Model file for the job. Use its own axes, mm. Face numbers are marked on the shaded views. A direction names the side the tool comes from. Round coordinates to 2 decimals unless told otherwise and drop trailing zeros. Order: outer loops, then holes, each group sorted by start corner. A loop starts at its lowest first (then second) coordinate and runs counter-clockwise, first axis right, second up. Notation, with made-up numbers: (25, -23) -> (30, -23) arc R15 ccw to (30, 3) -> close; hole circle Ø6 at (-20.5, 41.5). An arc over 180 degrees is marked (long way). Answer as CSV lines item,"result".
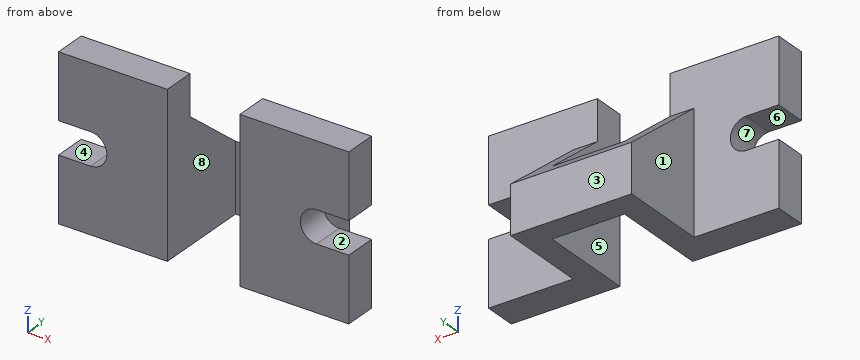
```python
from build123d import *

# Parameters (mm, degrees)
SKETCH_1_W               = 72
SKETCH_1_H               = 40
EXTRUDE_1_DEPTH          = 8
SKETCH_2_W               = 30
SKETCH_2_H               = 40
EXTRUDE_2_DEPTH          = 30
CUT_EXTRUDE_1_DEPTH      = 30
CUT_EXTRUDE_1_DEPTH_BACK = 30
CUT_EXTRUDE_2_DEPTH      = 30
CUT_EXTRUDE_2_DEPTH_BACK = 30
SKETCH_4_W               = 18
SKETCH_4_H               = 24
CUT_EXTRUDE_4_DEPTH      = 30
CUT_EXTRUDE_4_DEPTH_BACK = 30


with BuildPart() as part:
    # 草图1 → 凸台-拉伸1 (new body)
    with BuildSketch(Plane(origin=(0, 0, 0), x_dir=(1, 0, 0), z_dir=(0, 1, 0))):
        Rectangle(SKETCH_1_W, SKETCH_1_H)
    extrude(amount=EXTRUDE_1_DEPTH)

    # 草图2 → 凸台-拉伸2 (add)
    with BuildSketch(Plane(origin=(0, 0, 0), x_dir=(1, 0, 0), z_dir=(0, 1, 0))):
        Rectangle(SKETCH_2_W, SKETCH_2_H)
    extrude(amount=EXTRUDE_2_DEPTH)

    # 草图3 → 切除-拉伸1 (cut, two sides: drawn at the far end of the back side and taken through both)
    with BuildSketch(Plane(origin=(0, 0, 0), x_dir=(0, 0, -1), z_dir=(1, 0, 0)).offset(-CUT_EXTRUDE_1_DEPTH_BACK)):
        Polygon((-9.996476923, 8), (8, 30), (-20, 30), (-20, 8), align=None)
    extrude(amount=CUT_EXTRUDE_1_DEPTH + CUT_EXTRUDE_1_DEPTH_BACK, mode=Mode.SUBTRACT)

    # 草图4 → 切除-拉伸2 (cut, two sides: drawn at the far end of the back side and taken through both)
    with BuildSketch(Plane.XY.offset(-CUT_EXTRUDE_2_DEPTH_BACK)):
        with Locations((0, 12)):
            Rectangle(SKETCH_4_W, SKETCH_4_H)
    extrude(amount=CUT_EXTRUDE_2_DEPTH + CUT_EXTRUDE_2_DEPTH_BACK, mode=Mode.SUBTRACT)

    # 草图7 → 切除-拉伸4 (cut, two sides: drawn at the far end of the back side and taken through both)
    with BuildSketch(Plane(origin=(0, 0, 0), x_dir=(1, 0, 0), z_dir=(0, 1, 0)).offset(-CUT_EXTRUDE_4_DEPTH_BACK)):
        with BuildLine():
            Line((-28, 4), (-36, 4))
            Line((-36, 4), (-36, -4))
            Line((-36, -4), (-28, -4))
            ThreePointArc((-28, -4), (-24, 0), (-28, 4))
        make_face()
        with BuildLine():
            Line((28, 4), (36, 4))
            Line((36, 4), (36, -4))
            Line((36, -4), (28, -4))
            ThreePointArc((28, -4), (24, 0), (28, 4))
        make_face()
    extrude(amount=CUT_EXTRUDE_4_DEPTH + CUT_EXTRUDE_4_DEPTH_BACK, mode=Mode.SUBTRACT)


solid = part.part
```
Q1. Saw through at C-C (z = 8). Write the cut outline in (x, y), plus the area to 3 significant figures.
Checks:
outline,"(-36, 0) -> (-9, 0) -> (-9, 10.44) -> (-15, 10.44) -> (-15, 8) -> (-36, 8) -> close; (9, 0) -> (36, 0) -> (36, 8) -> (15, 8) -> (15, 10.44) -> (9, 10.44) -> close"
area,"461 mm²"
Q2. Saw through at A-A (y = 5.5). Write the cut outline in (x, z), plus the area to 3 significant figures.
Checks:
outline,"(-36, -20) -> (-9, -20) -> (-9, 20) -> (-36, 20) -> (-36, 4) -> (-28, 4) arc R4 cw to (-28, -4) -> (-36, -4) -> close; (9, -20) -> (36, -20) -> (36, -4) -> (28, -4) arc R4 cw to (28, 4) -> (36, 4) -> (36, 20) -> (9, 20) -> close"
area,"1,980 mm²"
Q3. Saw through at B-B (x = -31). Write the cut outline in (y, z).
Checks:
outline,"(0, -20) -> (8, -20) -> (8, -4) -> (0, -4) -> close; (0, 4) -> (8, 4) -> (8, 20) -> (0, 20) -> close"
Q4. Flat gauge pins, fed straight in: pin 1 (17.5 mm diameter, centred on y = 22, z = -4.5, fed in from -X); pin 2 (5 mm diameter, centred on x = -13.5, z = 16, fed in from +Y); pin 3 (1 mm diameter, centred on x = 10.5, z = 1.5, fed in from +Y). Where does each tip first touch, or does it go through?
Checks:
pin 1,"x = -15"
pin 2,"y = 8"
pin 3,"y = 19"
Q5. Mould opens along X. For the marked faces 6, 7 and 8 say: +X half, -X half, draft (parallel to the pull), parting line (faces both ways), or undercut.
Checks:
face 6,"draft"
face 7,"-X half"
face 8,"undercut"
Q6. Wall check: L1, parallel to X at y = 18.5, z = -16.5; L2, parallel to X at y = 4.5, z = 11.5; L3, parallel to Y at x = 26.5, z = -16. Give the ranges that are in metal, low to high. Write a range as [from, to].
Checks:
L1,"[-15, -9], [9, 15]"
L2,"[-36, -9], [9, 36]"
L3,"[0, 8]"
Q7. Saw through at D-D (z = -15). Write the cut outline in (x, y).
Checks:
outline,"(-36, 0) -> (-9, 0) -> (-9, 24) -> (9, 24) -> (9, 0) -> (36, 0) -> (36, 8) -> (15, 8) -> (15, 30) -> (-15, 30) -> (-15, 8) -> (-36, 8) -> close"
Q8. Tool access for the marked faces 1, 2, 3, 4 and 5: list every direction of +Z, -Z, +X, -X, +Y, -Y with a clear straight run to the whole face (end or side of a thin tool).
Checks:
face 1,"+Z, -Z, -X, +Y"
face 2,"+X, +Y, -Y"
face 3,"+Z, -Z, +X, -X, +Y"
face 4,"-X, +Y, -Y"
face 5,"+Z, -Z, -Y"
